Autodesk Inventor part; units mm, degrees
ref_plane "YZ Plane" through (0, 0, 0) normal (1, 0, 0) x (0, 1, 0)
ref_plane "XZ Plane" through (0, 0, 0) normal (0, 1, 0) x (-1, 0, 0)
ref_plane "XY Plane" through (0, 0, 0) normal (0, 0, 1) x (1, 0, 0)
sketch "스케치1" plane through (0, 0, 0) normal (0, 0, 1) x (1, 0, 0)
  circle A0 centre (0, 0) radius 11
  circle A1 centre (0, -8) radius 1.1
  circle A2 centre (0, 0) radius 11
  circle A3 centre (8, 0) radius 1.1
  circle A4 centre (0, 0) radius 11
  circle A5 centre (0, 8) radius 1.1
  circle A6 centre (0, 0) radius 11
  circle A7 centre (-8, 0) radius 1.1
  arc A8 (-11, 0) -> (11, 0) centre (0, 0) ccw
  circle A9 centre (0, 0) radius 4.5
  line L0 (0, 11) -> (30, 11)
  line L1 (30, 11) -> (30, -11)
  line L2 (30, -11) -> (0, -11)
  arc A10 (0, -11) -> (0, 11) centre (0, 0) ccw
  dimension "d2" = 2.2
  dimension "d3" = 360
  dimension "d4" = 9
  dimension "d5" = 30
extrude "돌출1" add sketch "스케치1" along normal blind 5
sketch "스케치7" plane through (30, -11, 0) normal (1, 0, 0) x (0, 0, -1)
  line L0 (0, 0) -> (-5, 0)
  line L1 (0, 22) -> (-5, 22)
  line L2 (0, 0) -> (-5, 0)
  line L3 (-5, 0) -> (-5, 22)
  line L4 (-5, 22) -> (0, 22)
  line L5 (0, 22) -> (0, 0)
  point P0 (0, 11)
sketch "스케치8" plane through (0, -11, 0) normal (0, -1, 0) x (1, 0, 0)
  line L0 (30, 0) -> (0, 0)
  arc A0 (70, -40) -> (30, 0) centre (30, -40) ccw
  line L1 (30, -40) -> (70, -40) construction
  line L2 (30, -40) -> (30, 0) construction
  arc A1 (90, -60) -> (30, 0) centre (30, -60) ccw
  line L3 (30, -60) -> (90, -60) construction
  line L4 (30, -60) -> (30, 0) construction
  dimension "d13" = 90
  dimension "d29" = 90
sweep "스윕2" add profiles "스케치7" path "스케치8" path curves A1
sketch "스케치9" plane through (75, -11, -60) normal (0, 0, -1) x (-1, 0, 0)
  line L0 (45, 0) -> (5, 0)
  line L1 (5, 22) -> (0, 22)
  line L2 (-14.9739, 0) -> (-19.9739, 0)
  line L3 (-19.9739, 0) -> (-19.9739, 22)
  line L4 (-19.9739, 22) -> (-14.9739, 22)
  line L5 (-14.9739, 22) -> (-14.9739, 0)
  point P0 (75, 11)
extrude "돌출3" add sketch "스케치9" along normal blind 30
sketch "스케치10" plane through (94.9739, -11, -40) normal (1, 0, 0) x (0, 0, -1)
  line L0 (50, 0) -> (50, 22)
  circle A0 centre (50, 11) radius 11
  circle A1 centre (50, 11) radius 4.5
  circle A2 centre (50, 3) radius 1.1
  circle A3 centre (58, 11) radius 1.1
  circle A4 centre (50, 19) radius 1.1
  circle A5 centre (42, 11) radius 1.1
  point P0 (-40, 11)
  dimension "d18" = 9
  dimension "d19" = 2.2
  dimension "d20" = 8
  dimension "d23" = 360
extrude "돌출4" add sketch "스케치10" against normal blind 5 contours A0 L0 A4 A1 A2 | L0 A2 A1 A4 A0
extrude "돌출5" cut sketch "스케치10" against normal blind 5 contours A2 L0 | L0 A2 | A4 L0 | L0 A4 | A1 L0 | L0 A1 | A5
sketch "스케치11" plane through (89.9739, -11, -60) normal (-1, 0, 0) x (0, 0, 1)
  circle A0 centre (-30, 3) radius 1.1
  circle A1 centre (-30, 3) radius 2.1
  circle A2 centre (-22, 11) radius 1.1
  circle A3 centre (-22, 11) radius 2.1
  circle A4 centre (-38, 11) radius 1.1
  circle A5 centre (-38, 11) radius 2.1
  circle A6 centre (-30, 19) radius 1.1
  circle A7 centre (-30, 19) radius 2.1
  point P0 (60, 11)
  dimension "d30" = 4.2
  dimension "d31" = 4.2
  dimension "d32" = 4.2
  dimension "d33" = 4.2
sketch "스케치12" plane through (0, 0, 0) normal (0, 0, -1) x (-1, 0, 0)
  circle A0 centre (0, -8) radius 1.1
  circle A1 centre (0, -8) radius 2.1
  circle A2 centre (8, 0) radius 1.1
  circle A3 centre (8, 0) radius 2.1
  circle A4 centre (-8, 0) radius 1.1
  circle A5 centre (-8, 0) radius 2.1
  circle A6 centre (0, 8) radius 1.1
  circle A7 centre (0, 8) radius 2.1
  point P0 (0, 0)
  dimension "d34" = 4.2
  dimension "d35" = 4.2
  dimension "d36" = 4.2
  dimension "d37" = 4.2
extrude "돌출6" cut sketch "스케치11" against normal blind 3
extrude "돌출7" cut sketch "스케치12" against normal blind 3
properties part number "shoulder2"
Could you check a few things on this model? Use its own coordinates, in mm. A direction names the side the tool comes from. Give positions to 0.01 mm unless a question says otherwise; leave off trailing zeros. Order: outer loops, then holes, each group sorted by start corner. A loop starts at its lowest first (then second) coordinate and runs counter-clockwise, first axis right, second up.
1. Which directions (+Z, -Z, +X, -X, +Y, -Y) give clear straight access to the entire face, cutting with the end or side of a thin tool? Please do faces 1 (the cylindrical face through (0.273, 10.082, 1.479)), 2 (the cylindrical face through (91.45, -7.91, -92.1)), 3 (the flat face through (69, 11, -14)).
Answers below:
face 1: -Z
face 2: -X
face 3: +Z, -Z, +X, -X, +Y
2. Thinking about a two-plate mould opening in Z: for faces 4 (the cylindrical face through (-0.59, -4.46, 2.46)), 5 (the flat face through (14, 0, 5)), 6 (the flat face through (92.974, -1, -97)), which applies, +Z half, -Z half, draft (parallel to the pull), parting line (faces both ways), or undercut?
Answers below:
face 4: draft
face 5: +Z half
face 6: undercut
3. I need wall thicknesses on L1, parallel to Y at x = 0, z = 3.6; L2, parallel to Y at x = 91.95, z = -90; L3, parallel to Y at x = 94, z = -82. Which ranges of each line are inside material? Lowest first, please.
Answers below:
L1: y = -11 to -9.1, -6.9 to -4.5, 4.5 to 6.9, 9.1 to 11
L2: y = -11 to -10.1, -5.9 to -4.5, 4.5 to 5.9, 10.1 to 11
L3: y = -11 to -1.1, 1.1 to 11
4. Suppose I cut it at B-B (x = 69.5). Write out the boundary of the cut face in (y, z), plus the area to 3 significant figures.
Answers below:
outline: (-11, -14.84) - (11, -14.84) - (11, -8.38) - (-11, -8.38) - close
area: 142 mm2
5. For pin 1 (2.5 mm diameter, centred on y = 0, z = -82, fed in from -X); pin 2 (2.5 mm diameter, centred on y = 0, z = -98, fed in from +X); pin 3 (6 mm diameter, centred on x = 55, y = -4, fed in from +Z); pin 4 (5.5 mm diameter, centred on y = 0, z = -90, fed in from +X), each with a flat end and sliding along its axis, tell me the tip position at first contact or that it passes through.
Answers below:
pin 1: stops at x = 92.97
pin 2: stops at x = 94.97
pin 3: stops at z = 1.16
pin 4: passes through
6. Suppose I cut it at A-A (z = -66.5). Write out the boundary of the cut face in (x, y).
Answers below:
outline: (89.97, -11) - (94.97, -11) - (94.97, 11) - (89.97, 11) - close
